```python
from build123d import *

# Parameters (mm, degrees)
SKETCH1_W            = 81.28
SKETCH1_H            = 81.28
SKETCH1_W_2          = 76.2
SKETCH1_H_2          = 76.2
BOSS_EXTRUDE1_DEPTH  = 177.8
SKETCH2_W            = 2.54
SKETCH2_H            = 38.1
BOSS_EXTRUDE2_DEPTH  = 25.4
SKETCH3_W            = 2.54
SKETCH3_H            = 25.4
CUT_EXTRUDE1_DEPTH   = 212.720846399
BOSS_EXTRUDE3_DEPTH  = 12.7
BOSS_EXTRUDE4_DEPTH  = 12.7
SKETCH14_W           = 5.08
SKETCH14_H           = 25.4
BOSS_EXTRUDE6_DEPTH  = 76.2
CUT_EXTRUDE2_REACH   = 243.407
SKETCH16_W           = 24.13
SKETCH16_H           = 20.32
SKETCH22_R           = 2
CUT_EXTRUDE6_DEPTH   = 252.036309724
SKETCH28_W           = 25.4
SKETCH28_H           = 50.8
BOSS_EXTRUDE7_DEPTH  = 38.1
CUT_EXTRUDE8_REACH   = 245.43
SKETCH32_W           = 33.02
SKETCH32_H           = 20.32
CUT_EXTRUDE9_DEPTH   = 25.4
CUT_EXTRUDE13_REACH  = 245.27
SKETCH34_R           = 8.89
BOSS_EXTRUDE9_DEPTH  = 2.54
SKETCH38_W           = 2.54
SKETCH38_H           = 25.4
CUT_EXTRUDE15_DEPTH  = 63.5
CUT_EXTRUDE17_REACH  = 224.71
SKETCH40_R           = 2.5
SKETCH41_R           = 3.77
SKETCH41_R_2         = 2.5
BOSS_EXTRUDE10_DEPTH = 5
SKETCH42_R           = 3.77
SKETCH42_R_2         = 2.5
BOSS_EXTRUDE11_DEPTH = 5
SKETCH43_W           = 76.2
SKETCH43_H           = 76.2
CUT_EXTRUDE20_DEPTH  = 25.4
SKETCH44_W           = 174.6
SKETCH44_H           = 70
SKETCH44_R           = 1.5
BOSS_EXTRUDE12_DEPTH = 2.54
BOSS_EXTRUDE13_DEPTH = 2.54
BOSS_EXTRUDE14_DEPTH = 2.54
BOSS_EXTRUDE15_REACH = 264.115
BOSS_EXTRUDE16_DEPTH = 2.54
BOSS_EXTRUDE17_DEPTH = 2.54
BOSS_EXTRUDE18_REACH = 264.115
SKETCH51_R           = 2
CUT_EXTRUDE21_DEPTH  = 2.54


with BuildPart() as part:
    # Sketch1 → Boss-Extrude1 (new body)
    with BuildSketch(Plane(origin=(0, 0, 0), x_dir=(1, 0, 0), z_dir=(0, 1, 0))):
        with Locations((40.64, 40.64)):
            Rectangle(SKETCH1_W, SKETCH1_H)
        with Locations((40.64, 40.64)):
            Rectangle(SKETCH1_W_2, SKETCH1_H_2, mode=Mode.SUBTRACT)
    extrude(amount=BOSS_EXTRUDE1_DEPTH)

    # Sketch2 → Boss-Extrude2 (add)
    with BuildSketch(Plane(origin=(0, 0, 0), x_dir=(0, 0, -1), z_dir=(1, 0, 0))):
        with Locations((64.77, 19.05)):
            Rectangle(SKETCH2_W, SKETCH2_H)
    extrude(amount=-BOSS_EXTRUDE2_DEPTH)

    # Sketch3 → Cut-Extrude1 (cut, through all)
    with BuildSketch(Plane.XY):
        with Locations((80.01, 12.7)):
            Rectangle(SKETCH3_W, SKETCH3_H)
    extrude(amount=-CUT_EXTRUDE1_DEPTH, mode=Mode.SUBTRACT)

    # Sketch7 → Boss-Extrude3 (add)
    with BuildSketch(Plane.XY):
        Polygon((81.28, 25.4), (106.68, 50.8), (81.28, 50.8), align=None)
    extrude(amount=-BOSS_EXTRUDE3_DEPTH)

    # Sketch10 → Boss-Extrude4 (add)
    with BuildSketch(Plane(origin=(0, 0, -81.28), x_dir=(-1, 0, 0), z_dir=(0, 0, -1))):
        Polygon((-81.28, 25.4), (-81.28, 50.8), (-106.68, 50.8), align=None)
    extrude(amount=-BOSS_EXTRUDE4_DEPTH)

    # Sketch14 → Boss-Extrude6 (add)
    with BuildSketch(Plane(origin=(81.28, 0, 0), x_dir=(0, 0, -1), z_dir=(1, 0, 0))):
        with Locations((40.64, 38.1)):
            Rectangle(SKETCH14_W, SKETCH14_H)
    extrude(amount=BOSS_EXTRUDE6_DEPTH)

    # Sketch16 → Cut-Extrude2 (cut, up to next)
    with BuildSketch(Plane.XY.offset(-38.1), mode=Mode.PRIVATE) as cut_extrude2_sk1:
        with Locations((128.905, 40.64)):
            Rectangle(SKETCH16_W, SKETCH16_H)
    cut_extrude2_tool1 = extrude(cut_extrude2_sk1.sketch, amount=-CUT_EXTRUDE2_REACH, mode=Mode.PRIVATE) & part.part
    add(cut_extrude2_tool1.solids().sort_by_distance((128.905, 40.64, -38.1))[0], mode=Mode.SUBTRACT)

    # Sketch22 → Cut-Extrude6 (cut, through all)
    with BuildSketch(Plane.XY):
        with Locations((93.98, 45.72)):
            Circle(SKETCH22_R)
    extrude(amount=-CUT_EXTRUDE6_DEPTH, mode=Mode.SUBTRACT)

    # Sketch28 → Boss-Extrude7 (add)
    with BuildSketch(Plane(origin=(81.28, 0, 0), x_dir=(0, 0, -1), z_dir=(1, 0, 0))):
        with Locations((40.64, 152.4)):
            Rectangle(SKETCH28_W, SKETCH28_H)
    extrude(amount=BOSS_EXTRUDE7_DEPTH)

    # Sketch30 → Cut-Extrude8 (cut, up to next)
    with BuildSketch(Plane.XY.offset(-27.94), mode=Mode.PRIVATE) as cut_extrude8_sk1:
        Polygon((81.28, 127), (119.38, 127), (119.38, 152.4), align=None)
    cut_extrude8_tool1 = extrude(cut_extrude8_sk1.sketch, amount=-CUT_EXTRUDE8_REACH, mode=Mode.PRIVATE) & part.part
    add(cut_extrude8_tool1.solids().sort_by_distance((106.68, 135.466667, -27.94))[0], mode=Mode.SUBTRACT)

    # Sketch32 → Cut-Extrude9 (cut)
    with BuildSketch(Plane(origin=(0, 177.8, 0), x_dir=(1, 0, 0), z_dir=(0, 1, 0))):
        with Locations((100.33, 40.64)):
            Rectangle(SKETCH32_W, SKETCH32_H)
    extrude(amount=-CUT_EXTRUDE9_DEPTH, mode=Mode.SUBTRACT)

    # Cut-Extrude13: up to this face of the body (flat: up to its plane)
    cut_extrude13_end = Plane(part.part.faces().sort_by_distance((78.74, 101.6, -40.64))[0])
    # Sketch34 → Cut-Extrude13 (cut, up to the picked face)
    with BuildSketch(Plane(origin=(119.38, 0, 0), x_dir=(0, 0, -1), z_dir=(1, 0, 0)), mode=Mode.PRIVATE) as cut_extrude13_sk1:
        with Locations(Location((40.64, 165.1, 0), (0, 0, 180))):
            Circle(SKETCH34_R)
    cut_extrude13_tool1 = split(extrude(cut_extrude13_sk1.sketch, amount=-CUT_EXTRUDE13_REACH, mode=Mode.PRIVATE), bisect_by=cut_extrude13_end, keep=Keep.BOTH, mode=Mode.PRIVATE)
    add(cut_extrude13_tool1.solids().sort_by(Axis((119.38, 165.1, -40.64), (-1, 0, 0)))[0], mode=Mode.SUBTRACT)

    # Sketch37 → Boss-Extrude9 (add)
    with BuildSketch(Plane.XY.offset(-63.5)):
        Polygon((-25.4, 38.1), (0, 38.1), (0, 52.764696837), align=None)
    extrude(amount=-BOSS_EXTRUDE9_DEPTH)

    # Sketch38 → Cut-Extrude15 (cut)
    with BuildSketch(Plane.XY):
        with Locations((1.27, 12.7)):
            Rectangle(SKETCH38_W, SKETCH38_H)
    extrude(amount=-CUT_EXTRUDE15_DEPTH, mode=Mode.SUBTRACT)

    # Cut-Extrude17: up to this face of the body (flat: up to its plane)
    cut_extrude17_end = Plane(part.part.faces().sort_by_distance((0, 99.23335202, -41.514066738))[0])
    # Sketch40 → Cut-Extrude17 (cut, up to the picked face)
    with BuildSketch(Plane(origin=(81.28, 0, 0), x_dir=(0, 0, -1), z_dir=(1, 0, 0)), mode=Mode.PRIVATE) as cut_extrude17_sk1:
        with Locations((19.05, 101.6)):
            Circle(SKETCH40_R)
    cut_extrude17_tool1 = split(extrude(cut_extrude17_sk1.sketch, amount=-CUT_EXTRUDE17_REACH, mode=Mode.PRIVATE), bisect_by=cut_extrude17_end, keep=Keep.BOTH, mode=Mode.PRIVATE)
    # Sketch40 → Cut-Extrude17 (cut, up to the picked face)
    with BuildSketch(Plane(origin=(81.28, 0, 0), x_dir=(0, 0, -1), z_dir=(1, 0, 0)), mode=Mode.PRIVATE) as cut_extrude17_sk2:
        with Locations((62.23, 101.6)):
            Circle(SKETCH40_R)
    cut_extrude17_tool2 = split(extrude(cut_extrude17_sk2.sketch, amount=-CUT_EXTRUDE17_REACH, mode=Mode.PRIVATE), bisect_by=cut_extrude17_end, keep=Keep.BOTH, mode=Mode.PRIVATE)
    add(cut_extrude17_tool1.solids().sort_by(Axis((81.28, 101.6, -19.05), (-1, 0, 0)))[0], mode=Mode.SUBTRACT)
    add(cut_extrude17_tool2.solids().sort_by(Axis((81.28, 101.6, -62.23), (-1, 0, 0)))[0], mode=Mode.SUBTRACT)

    # Sketch41 → Boss-Extrude10 (add)
    with BuildSketch(Plane(origin=(81.28, 0, 0), x_dir=(0, 0, -1), z_dir=(1, 0, 0))):
        with Locations(Location((19.05, 101.6, 0), (0, 0, 180))):
            Circle(SKETCH41_R)
        with Locations((19.05, 101.6)):
            Circle(SKETCH41_R_2, mode=Mode.SUBTRACT)
        with Locations(Location((62.23, 101.6, 0), (0, 0, 180))):
            Circle(SKETCH41_R)
        with Locations((62.23, 101.6)):
            Circle(SKETCH41_R_2, mode=Mode.SUBTRACT)
    extrude(amount=BOSS_EXTRUDE10_DEPTH)

    # Sketch42 → Boss-Extrude11 (add)
    with BuildSketch(Plane.ZY):
        with Locations((-62.23, 101.6)):
            Circle(SKETCH42_R)
        with Locations(Location((-62.23, 101.6, 0), (0, 0, 180))):
            Circle(SKETCH42_R_2, mode=Mode.SUBTRACT)
        with Locations((-19.05, 101.6)):
            Circle(SKETCH42_R)
        with Locations(Location((-19.05, 101.6, 0), (0, 0, 180))):
            Circle(SKETCH42_R_2, mode=Mode.SUBTRACT)
    extrude(amount=BOSS_EXTRUDE11_DEPTH)

    # Sketch43 → Cut-Extrude20 (cut)
    with BuildSketch(Plane(origin=(0, 177.8, 0), x_dir=(1, 0, 0), z_dir=(0, 1, 0))):
        Polygon((83.82, 53.34), (83.82, 27.94), (81.28, 27.94), (81.28, 0), (0, 0), (0, 81.28), (81.28, 81.28), (81.28, 53.34), align=None)
        with Locations((40.64, 40.64)):
            Rectangle(SKETCH43_W, SKETCH43_H, mode=Mode.SUBTRACT)
    extrude(amount=-CUT_EXTRUDE20_DEPTH, mode=Mode.SUBTRACT)

    # Sketch44 → Boss-Extrude12 (add)
    with BuildSketch(Plane.XY):
        with Locations((87.3, 85.8)):
            Rectangle(SKETCH44_W, SKETCH44_H)
        with Locations((140.97, 115.8)):
            Circle(SKETCH44_R, mode=Mode.SUBTRACT)
        with Locations((140.97, 55.8)):
            Circle(SKETCH44_R, mode=Mode.SUBTRACT)
    extrude(amount=-BOSS_EXTRUDE12_DEPTH)

    # Sketch45 → Boss-Extrude13 (add)
    with BuildSketch(Plane.XY):
        Polygon((0, 152.4), (-25.4, 152.4), (0, 127), align=None)
    extrude(amount=-BOSS_EXTRUDE13_DEPTH)

    # Sketch46 → Boss-Extrude14 (add)
    with BuildSketch(Plane(origin=(0, 0, -81.28), x_dir=(-1, 0, 0), z_dir=(0, 0, -1))):
        Polygon((0, 152.4), (0, 127), (25.4, 152.4), align=None)
    extrude(amount=-BOSS_EXTRUDE14_DEPTH)

    # Sketch47 → Boss-Extrude15 (add, up to next)
    with BuildSketch(Plane.XY, mode=Mode.PRIVATE) as boss_extrude15_sk1:
        Polygon((0, 152.4), (-25.4, 152.4), (-22.86, 149.86), (0, 149.86), align=None)
    boss_extrude15_tool1 = extrude(boss_extrude15_sk1.sketch, amount=-BOSS_EXTRUDE15_REACH, mode=Mode.PRIVATE) - part.part
    add(boss_extrude15_tool1.solids().sort_by_distance((-12.07614, 151.152281, 0))[0])

    # Sketch48 → Boss-Extrude16 (add)
    with BuildSketch(Plane.XY):
        Polygon((81.28, 152.4), (106.68, 152.4), (81.28, 127), align=None)
    extrude(amount=-BOSS_EXTRUDE16_DEPTH)

    # Sketch49 → Boss-Extrude17 (add)
    with BuildSketch(Plane(origin=(0, 0, -81.28), x_dir=(-1, 0, 0), z_dir=(0, 0, -1))):
        Polygon((-81.28, 152.4), (-106.68, 152.4), (-81.28, 127), align=None)
    extrude(amount=-BOSS_EXTRUDE17_DEPTH)

    # Sketch50 → Boss-Extrude18 (add, up to next)
    with BuildSketch(Plane(origin=(0, 0, -81.28), x_dir=(-1, 0, 0), z_dir=(0, 0, -1)), mode=Mode.PRIVATE) as boss_extrude18_sk1:
        Polygon((-81.28, 152.4), (-106.68, 152.4), (-104.14, 149.86), (-81.28, 149.86), align=None)
    boss_extrude18_tool1 = extrude(boss_extrude18_sk1.sketch, amount=-BOSS_EXTRUDE18_REACH, mode=Mode.PRIVATE) - part.part
    add(boss_extrude18_tool1.solids().sort_by_distance((93.35614, 151.152281, -81.28))[0])
    add(boss_extrude18_tool1.solids().sort_by_distance((93.35614, 151.152281, -81.28))[1])

    # Sketch51 → Cut-Extrude21 (cut)
    with BuildSketch(Plane(origin=(0, 152.4, 0), x_dir=(1, 0, 0), z_dir=(0, 1, 0))):
        with Locations(Location((-12.7, 68.58, 0), (0, 0, 270))):
            Circle(SKETCH51_R)
        with Locations(Location((-12.7, 40.64, 0), (0, 0, 270))):
            Circle(SKETCH51_R)
        with Locations(Location((-12.7, 12.7, 0), (0, 0, 270))):
            Circle(SKETCH51_R)
        with Locations(Location((93.98, 68.58, 0), (0, 0, 270))):
            Circle(SKETCH51_R)
        with Locations(Location((93.98, 12.7, 0), (0, 0, 270))):
            Circle(SKETCH51_R)
    extrude(amount=-CUT_EXTRUDE21_DEPTH, mode=Mode.SUBTRACT)


solid = part.part
```
Input: part model. Units: mm. Frame: model coordinates. A direction names the side the tool comes from. Give positions to 0.01 mm unless a question says otherwise; leave off trailing zeros. Order: outer loops, then holes, each group sorted by start corner. A loop starts at its lowest first (then second) coordinate and runs counter-clockwise, first axis right, second up.
1. Mould query, pull axis Z, two halves, no side actions, for faces 1 (the flat face through (76, 77, 0)), 2 (the flat face through (-9, 141, -78.74)), 3 (the flat face through (149, 50.8, -41)), 4 (the cylindrical face through (83.74, 97.86, -19.54)). Classes: released by +Z, released by -Z, zero draft, split by the parting line, or undercut.
Derived:
face 1: released by +Z
face 2: undercut
face 3: zero draft
face 4: undercut
2. Material intervals for L1, parallel to Z at x = 5, y = 23; L2, parallel to X at y = 46, z = -68; L3, parallel to Z at x = -12, y = 151, sorted ascending.
Derived:
L1: z = -81.28 to -78.74, -2.54 to 0
L2: x = 0 to 2.54, 78.74 to 81.28
L3: z = -81.28 to -70.45, -66.71 to -42.51, -38.77 to -14.57, -10.83 to 0
3. Section C-C on x = 137. Return the cut outline in (y, z), and give its area (3 significant figures).
Derived:
outline: (25.4, -43.18) - (30.48, -43.18) - (30.48, -38.1) - (25.4, -38.1) - close; (50.8, -2.54) - (120.8, -2.54) - (120.8, 0) - (50.8, 0) - close
area: 204 mm2
4. Pin query (flat end, axial travel): pin 1 (3 mm diameter, centred on y = 142.5, z = -26.5, fed in from -X); pin 2 (10 mm diameter, centred on y = 41.5, z = -65.5, fed in from +X); pin 3 (3 mm diameter, centred on x = 0.5, z = -38.5, fed in from -Y). Return the tip coordinate at first contact, or that it passes through.
Derived:
pin 1: stops at x = 0
pin 2: stops at x = 101.32
pin 3: stops at y = 25.4
5. Reachability of faces 5 (the flat face through (116.84, 40, -41)), 6 (the flat face through (98.74, 144.46, -79.79)), 7 (the flat face through (-7, 144, -2.54)), 8 (the flat face through (78.74, 88, -40)) from +Z, -Z, +X, -X, +Y, -Y: full face, straight path, thin tool, end or side. Return the list, or none.
Derived:
face 5: +Z, -Z
face 6: -Z, +X
face 7: -X, -Y
face 8: +Y, -Y
6. Section A-A on x = 67. Return the cut outline in (y, z).
Derived:
outline: (0, -81.28) - (152.4, -81.28) - (152.4, -78.74) - (0, -78.74) - close; (0, -2.54) - (152.4, -2.54) - (152.4, 0) - (0, 0) - close
7. Section B-B on y = 165.1. Return the cut outline in (x, z).
Derived:
outline: (83.82, -53.34) - (119.38, -53.34) - (119.38, -49.53) - (116.84, -49.53) - (116.84, -50.8) - (83.82, -50.8) - close; (83.82, -30.48) - (116.84, -30.48) - (116.84, -31.75) - (119.38, -31.75) - (119.38, -27.94) - (83.82, -27.94) - close
